Here's how the part is built. I have some questions about the finished solid (model axes, mm). Face numbers are marked on the shaded views. Give positions to 0.01 mm unless a question says otherwise; leave off trailing zeros. Write each loop counter-clockwise with the first axis right and the second up, starting at its lowest first coordinate (ties: lowest second). Pieces come first, ordered by that corner, then holes. Notation, with made-up numbers: (52.5, 67) - (71.5, 67) arc R26 cw to (71.5, 99) - close; hole circle Ø7 at (70, -28). An arc over 180 degrees is marked (long way). Use a Markdown table: item, result.
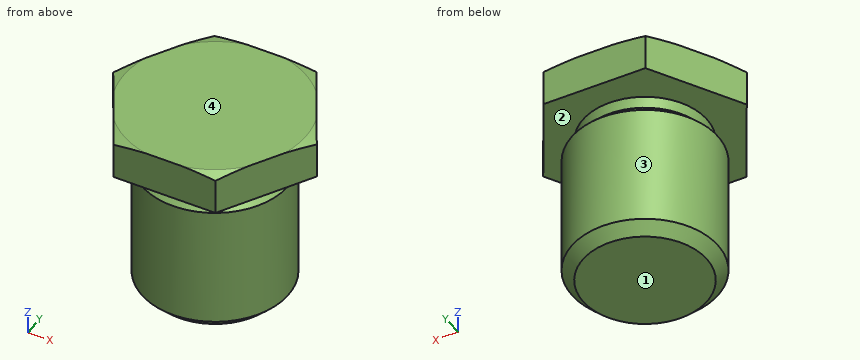
Autodesk Inventor part; units mm, degrees
ref_plane "YZ Plane" through (0, 0, 0) normal (1, 0, 0) x (0, 1, 0)
ref_plane "XZ Plane" through (0, 0, 0) normal (0, 1, 0) x (-1, 0, 0)
ref_plane "XY Plane" through (0, 0, 0) normal (0, 0, 1) x (1, 0, 0)
sketch "Szkic7" plane through (0, 0, 0) normal (0, 0, 1) x (1, 0, 0)
  circle A0 centre (0, 0) radius 6.5785
  dimension "d35" = 13.157
extrude "Wyciągnięcie proste2" add sketch "Szkic7" along normal mid plane 12.9062
chamfer "Faza2" distance 1 angle 45 1 edges at (-6.5785, 0, 6.4531)
sketch "Szkic9" plane through (0, 0, 6.4531) normal (0, 0, 1) x (1, 0, 0)
  circle A0 centre (0, 0) radius 5.5785
extrude "Wyciągnięcie proste3" add sketch "Szkic9" along normal blind 1.0938
sketch "Szkic10" plane through (0, 0, 7.5469) normal (0, 0, 1) x (1, 0, 0)
  line L0 (-4.6188, 8) -> (4.6188, 8)
  line L1 (4.6188, 8) -> (9.2376, 0)
  line L2 (9.2376, 0) -> (4.6188, -8)
  line L3 (4.6188, -8) -> (-4.6188, -8)
  line L4 (-4.6188, -8) -> (-9.2376, 0)
  line L5 (-9.2376, 0) -> (-4.6188, 8)
  line L6 (0, 9.2099) -> (0, -9.2099) construction
  line L7 (-9.6995, 0) -> (9.6995, 0) construction
  point P0 (0, 0)
  point P1 (0, 0)
  point P2 (0, 8)
  dimension "d44" = 16
extrude "Wyciągnięcie proste4" add sketch "Szkic10" along normal blind 3.5
sketch "Szkic12" plane through (0, 0, 0) normal (0, 1, 0) x (-1, 0, 0)
  line L0 (0, -2.1463) -> (0, 12.8775) construction
  line L1 (-4.6188, 7.5469) -> (-4.6188, 11.0469) construction
  line L2 (-9.2376, 11.0469) -> (-4.6188, 11.0469) construction
  line L3 (-9.2376, 7.5469) -> (-9.2376, 11.0469)
  line L4 (-9.2376, 10.7611) -> (-8.1709, 11.0469)
  line L5 (-9.2376, 11.0469) -> (-4.6188, 11.0469)
  line L6 (-9.2376, 7.5469) -> (-4.6188, 7.5469)
  point P0 (0, 0)
  dimension "d50" = 15
  dimension "d51" = 1.0667
revolve "Obrót2" cut sketch "Szkic12" angle 360 about axis through (0, 0, -10) along (0, 0, 1)
thread "Gwint3"
chamfer "Faza3" distance 1 angle 45 1 edges at (-6.5785, 0, -6.4531)
equation "\"d35\" = OD"
equation "\"d36\" = 0.7375 * L"
equation "\"d42\" = 0.0625 * L"
equation "\"d44\" = SW"
equation "\"d45\" = 0.2 * L"
equation "\"d51\" = 0.0666667 * SW"
equation "\"SzerokośćGięciaPodcięcia\" = Grubość"
equation "\"RozmiarPodcięciaNarożnika\" = 4 * Grubość"
equation "\"PromieńPrzejścia\" = PromieńGięcia"
equation "\"Rozmiar_promienia_Jacobiego\" = PromieńGięcia"
equation "\"Wielk_odstępu\" = Grubość"
equation "\"d2\" = PromieńGięcia"
equation "\"d23\" = PromieńGięcia"
equation "\"OD\" = 13.157"
equation "\"SW\" = 16"
equation "\"L\" = 17.5"
properties part number "Korek sześciokątny BSP 1/4'' L=17,5" material "304"
Item 1: If we section it at A-A, the plane z = 9.75: Write out the boundary of the cut face in (x, y), plus the area to 3 significant figures.
Values:
| item | result |
|---|---|
| outline | (-9.24, 0) - (-4.62, -8) - (4.62, -8) - (9.24, 0) - (4.62, 8) - (-4.62, 8) - close |
| area | 222 mm2 |
Item 2: If we section it at D-D, the plane x = -7.5: Write out the boundary of the cut face in (y, z), plus the area to 3 significant figures.
Values:
| item | result |
|---|---|
| outline | (-3.01, 7.55) - (3.01, 7.55) - (3.01, 11.05) - (-3.01, 11.05) - close |
| area | 21.1 mm2 |
Item 3: I need wall thicknesses on line 1 along Z through (x, y) = (8, -0.25); line 2 along Z through (x, y) = (-4, -4.75); line 3 along Z through (x, y) = (1, 6). Which ranges of each line are inside material? Lowest first, please. Write a range as [from, to].
Values:
| item | result |
|---|---|
| line 1 | z = [7.55, 11.05] |
| line 2 | z = [-5.82, 5.82], [7.55, 11.05] |
| line 3 | z = [-5.95, 5.95], [7.55, 11.05] |
Item 4: If we section it at B-B, the plane x = 0: Write out the boundary of the cut face in (y, z).
Values:
| item | result |
|---|---|
| outline | (-8, 7.55) - (-5.58, 7.55) - (-5.58, 6.45) - (-6.58, 5.45) - (-6.58, -5.45) - (-5.58, -6.45) - (5.58, -6.45) - (6.58, -5.45) - (6.58, 5.45) - (5.58, 6.45) - (5.58, 7.55) - (8, 7.55) - (8, 11.05) - (-8, 11.05) - close |
Item 5: If we section it at C-C, the plane z = 3.5: Write out the boundary of the cut face in (x, y), plus the area to 3 significant figures.
Values:
| item | result |
|---|---|
| outline | circle Ø13.16 at (0, 0) |
| area | 136 mm2 |
Item 6: Thinking about a two-plate mould opening in Z: for the marked faces 1, 2, 3 and 4, which applies, +Z half, -Z half, draft (parallel to the pull), parting line (faces both ways), or undercut?
Values:
| item | result |
|---|---|
| face 1 | -Z half |
| face 2 | undercut |
| face 3 | draft |
| face 4 | +Z half |
Item 7: Will these pins go through, and if not, where does the flat tip stop? pin 1 Ø3 at (x, z) = (2, 6) entering from -Y; pin 2 Ø6 at (y, z) = (-6, 9) entering from +X; pin 3 Ø2 at (x, z) = (3, 3) entering from +Y.
Values:
| item | result |
|---|---|
| pin 1 | stops at y = -6.55 |
| pin 2 | stops at x = 7.51 |
| pin 3 | stops at y = 6.27 |
